Input: dimensioned drawing with shaded views. Units: mm. Origin: part minimum x, y, z. A direction names the side the tool comes from. Coordinates: 2 decimals unless noted, no trailing zeros. Loops run counter-clockwise (first coordinate to the right, second up) from the corner with the lowest first, then second, coordinate; pieces in that order, holes last. Notation, with made-up numbers: (-31, -23) -> (12, -23) arc R7 cw to (12, -18) -> close; hole circle Ø6 at (-32, 35). An arc over 180 degrees is marked (long way). Answer as CSV lines item,"result".
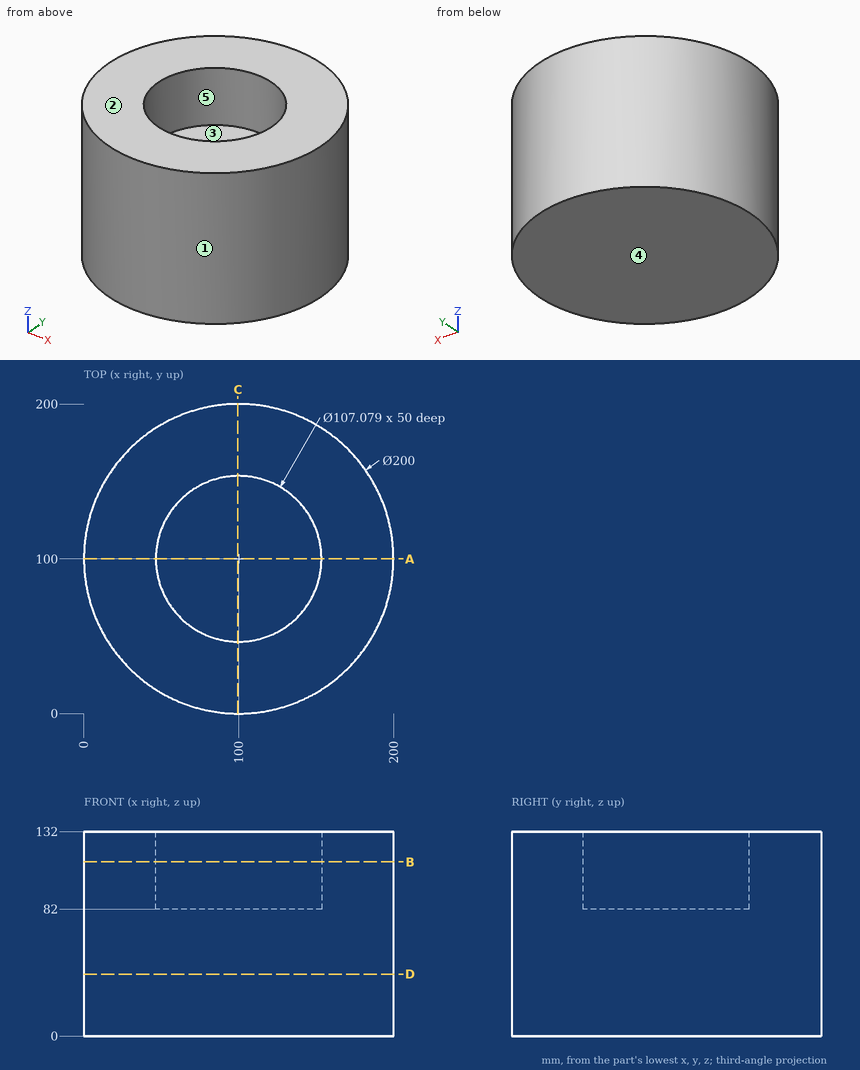
(1) Draft query along X for the marked faces 1, 2 and 3. Return one class per face: released by +X, released by -X, zero draft, split by the parting line, or undercut.
Computed values:
face 1,"split by the parting line"
face 2,"zero draft"
face 3,"undercut"
(2) Pin query (flat end, axial travel): pin 1 Ø3 at (x, z) = (20.5, 104.5) entering from +Y; pin 2 Ø10 at (x, y) = (121, 107.5) entering from +Z; pin 3 Ø12 at (y, z) = (26.5, 61) entering from +X. Return the tip coordinate at first contact, or that it passes through.
Computed values:
pin 1,"y = 162.58"
pin 2,"z = 82"
pin 3,"x = 173.78"
(3) Cut plane A-A (y = 100). Return the cut outline in (x, z).
Computed values:
outline,"(0, 0) -> (200, 0) -> (200, 132) -> (153.54, 132) -> (153.54, 82) -> (46.46, 82) -> (46.46, 132) -> (0, 132) -> close"
(4) Access query for the marked faces 4 and 5. Directions: +Z, -Z, +X, -X, +Y, -Y. A direction counts if a zero-diameter tool reaches every point of the face in a straight line with its end or side. Return the directions, or none.
Computed values:
face 4,"-Z, +X, -X, +Y, -Y"
face 5,"+Z"
(5) Material intervals for L1, parallel to Y at x = 100, z = 108; L2, parallel to X at y = 141.5, z = 120; L3, parallel to Z at x = 74, y = 127.5, sorted ascending. Write a range as [from, to].
Computed values:
L1,"[0, 46.46], [153.54, 200]"
L2,"[9.02, 66.17], [133.83, 190.98]"
L3,"[0, 82]"
(6) Cut plane D-D (z = 40). Return the cut outline in (x, y).
Computed values:
outline,"circle Ø200 at (100, 100)"
(7) Cut plane B-B (z = 112.5). Return the cut outline in (x, y), then the cut area to 3 significant figures.
Computed values:
outline,"circle Ø200 at (100, 100); hole circle Ø107.08 at (100, 100)"
area,"22,400 mm^2"
